```python
from build123d import *

# Parameters (mm, degrees)
F0_R     = 1.5
F0_R_2   = 2
F1_DEPTH = 3.2


with BuildPart() as f1:
    # F0 (on Front) → F1 (new body)
    with BuildSketch(Plane.XZ):
        with BuildLine():
            Line((3, -34), (3, 6))
            ThreePointArc((3, 6), (2.707107, 6.707107), (2, 7))
            Line((2, 7), (-2, 7))
            ThreePointArc((-2, 7), (-2.707107, 6.707107), (-3, 6))
            Line((-3, 6), (-3, -34))
            ThreePointArc((-3, -34), (-2.707107, -34.707107), (-2, -35))
            Line((-2, -35), (2, -35))
            ThreePointArc((2, -35), (2.707107, -34.707107), (3, -34))
        make_face()
        with Locations((0, -30.5)):
            Circle(F0_R, mode=Mode.SUBTRACT)
        with BuildLine():
            ThreePointArc((-2, -10), (0, -8), (2, -10))
            Line((2, -10), (2, -12))
            ThreePointArc((2, -12), (0, -14), (-2, -12))
            Line((-2, -12), (-2, -10))
        make_face(mode=Mode.SUBTRACT)
        Circle(F0_R_2, mode=Mode.SUBTRACT)
    extrude(amount=F1_DEPTH)


solid = f1.part
```
The model under review builds one solid part; all positions refer to its coordinate system, in mm. A direction names the side the tool comes from. Give positions to 0.01 mm unless a question says otherwise; leave off trailing zeros. Write each loop counter-clockwise with the first axis right and the second up, starting at its lowest first coordinate (ties: lowest second). Pieces come first, ordered by that corner, then holes. Notation, with made-up numbers: (50, 20) -> (84, 20) arc R32 cw to (84, 46) -> close; hole circle Ø1 at (8, 44.25). An arc over 180 degrees is marked (long way). Answer in a Markdown table with one row per item.
1) Add section C-C on x = 0.25. State the section outline as (y, z) points.
Worked answers:
| item | result |
|---|---|
| outline | (-3.2, -35) -> (0, -35) -> (0, -31.98) -> (-3.2, -31.98) -> close; (-3.2, -29.02) -> (0, -29.02) -> (0, -13.98) -> (-3.2, -13.98) -> close; (-3.2, -8.02) -> (0, -8.02) -> (0, -1.98) -> (-3.2, -1.98) -> close; (-3.2, 1.98) -> (0, 1.98) -> (0, 7) -> (-3.2, 7) -> close |
2) Add section B-B on z = -30.5. State the section outline as (x, y) points.
Worked answers:
| item | result |
|---|---|
| outline | (-3, -3.2) -> (-1.5, -3.2) -> (-1.5, 0) -> (-3, 0) -> close; (1.5, -3.2) -> (3, -3.2) -> (3, 0) -> (1.5, 0) -> close |
3) Mouldability with a two-part tool opening along X and no side actions: class faces 3 (the cylindrical face through (2.715, -1.578, 6.699)), 4 (the cylindrical face through (0, -2, -8)), 5 (the cylindrical face through (-2.715, -1.578, -34.699)) as +X half, -X half, draft (parallel to the pull), parting line (faces both ways), or undercut.
Worked answers:
| item | result |
|---|---|
| face 3 | +X half |
| face 4 | undercut |
| face 5 | -X half |
4) Add section A-A on y = -1.15. State the section outline as (x, z) points, plus the area to 3 significant figures.
Worked answers:
| item | result |
|---|---|
| outline | (-3, -34) arc R1 ccw to (-2, -35) -> (2, -35) arc R1 ccw to (3, -34) -> (3, 6) arc R1 ccw to (2, 7) -> (-2, 7) arc R1 ccw to (-3, 6) -> close; hole (-2, -12) arc R2 ccw to (2, -12) -> (2, -10) arc R2 ccw to (-2, -10) -> close; hole circle Ø4 at (0, 0); hole circle Ø3 at (0, -30.5) |
| area | 211 mm² |
5) Tool access review of faces 1 (the flat face through (-1, 0, -14)), 2 (the cylindrical face through (0, -2, -14)): name each direction out of +Z, -Z, +X, -X, +Y, -Y from which nothing blocks a thin tool from reaching the whole face with its end or side.
Worked answers:
| item | result |
|---|---|
| face 1 | +Z, -Z, +X, -X, +Y |
| face 2 | +Y, -Y |
6) For L1, parallel to Z at x = 0, y = -1.8; L2, parallel to Z at x = 1.25, y = -1.55; L3, parallel to X at y = -2.8, z = -13.5, list the stretches that pass through material, from the lowest coordinate up. Write a range as [from, to].
Worked answers:
| item | result |
|---|---|
| L1 | [-35, -32], [-29, -14], [-8, -2], [2, 7] |
| L2 | [-35, -31.33], [-29.67, -13.56], [-8.44, -1.56], [1.56, 7] |
| L3 | [-3, -1.32], [1.32, 3] |
